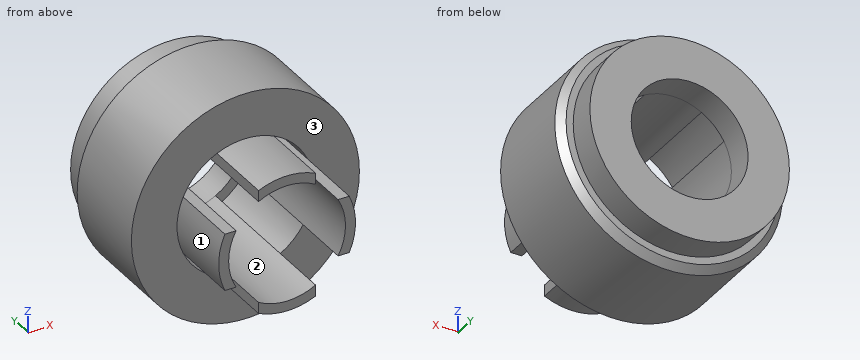
Autodesk Inventor part; units mm, degrees
ref_plane "YZ Plane" through (0, 0, 0) normal (1, 0, 0) x (0, 1, 0)
ref_plane "XZ Plane" through (0, 0, 0) normal (0, 1, 0) x (-1, 0, 0)
ref_plane "XY Plane" through (0, 0, 0) normal (0, 0, 1) x (1, 0, 0)
sketch "Sketch1" plane through (0, 0, 0) normal (0, 1, 0) x (-1, 0, 0)
  circle A0 centre (0, 0) radius 2.4
  circle A1 centre (0, 0) radius 4
  dimension "d0" = 8
  dimension "d1" = 4.8
extrude "Extrusion1" add sketch "Sketch1" along normal blind 3.5
chamfer "Chamfer1" distance 0.25 angle 45 1 edges at (4, 3.5, 0)
sketch "Sketch2" plane through (0, 3.5, 0) normal (0, 1, 0) x (1, 0, 0)
  circle A0 centre (0, 0) radius 2.05
  circle A1 centre (0, 0) radius 3.5
  dimension "d7" = 4.1
  dimension "d8" = 7
extrude "Extrusion2" add sketch "Sketch2" along normal blind 1
sketch "Sketch3" plane through (0, 3.5, 0) normal (0, -1, 0) x (1, 0, 0)
  arc A0 (-1.0733, -2.1466) -> (1, -2.1817) centre (0, 0) ccw
  arc A1 (-1, -1.7896) -> (1, -1.7896) centre (0, 0) ccw
  line L0 (-1, -1.7896) -> (-1, -2.1817)
  line L1 (1, -1.7896) -> (1, -2.1817)
  line L2 (0, 0) -> (0, -5.6159) construction
  dimension "d11" = 2.05
  dimension "d13" = 2.4
  dimension "d14" = 2
extrude "Extrusion3" add sketch "Sketch3" along normal blind 6
pattern_circular "Circular Pattern1" count 4 over 360 about axis through (0, -10, 0) along (0, 1, 0) of "Extrusion3"
properties part number "Collet" material "Acetal Resin, Black"
Part model, mm, in its own coordinate system. Face numbers are marked on the shaded views. A direction names the side the tool comes from. Coordinates: 2 decimals unless noted, no trailing zeros. Loops run counter-clockwise (first coordinate to the right, second up) from the corner with the lowest first, then second, coordinate; pieces in that order, holes last. Notation, with made-up numbers: M 45.5,81 L 70.5,81 A17 cw 70.5,87 Z; hole C 37,-19 d5. An arc over 180 degrees is marked long. Use a Markdown table: item, result. Add a question column.
Q1. Cut at A-A (y = -0.75). Write the cut outline in (x, z).
Q2. Pin check, flat tips, straight feed: P1, Ø1.5, axis at x = 3, y = 1, coming from the +Z side; P2, Ø2, axis at x = -1, y = 1, coming from the -Z side; P3, Ø0.9, axis at x = -1.5, z = 1.5, coming from the -Y side; P4, Ø1.5, axis at x = 0, y = -1.5, coming from the -Z side. Stop position of each tip, or through.
Q3. Cut at B-B (z = 0). Write the cut outline in (x, y), and give its area (3 significant figures).
Q4. Cut at C-C (x = 0). Write the cut outline in (y, z), and give its area (3 significant figures).
Q5. Probe L1, parallel to X at y = 4, z = 0; L2, parallel to X at y = -1.5, z = 0. List the from-to ranges inside material, lowest first.
Q6. Which spindle directions (+Z, -Z, +X, -X, +Y, -Y) get a long thin tool onto all of the face, cutting with end or side? Do the marked faces 1, 2 and 3. Say none if no direction does.
Q7. Cut at D-D (y = 1). Write the cut outline in (x, z), and give its area (3 significant figures).
Worked out:
| question | item | result |
|---|---|---|
| 1 | outline | M -2.18,-1 L -1.79,-1 A2.05 cw -1.79,1 L -2.18,1 A2.4 ccw Z; M -1,-2.18 A2.4 ccw 1,-2.18 L 1,-1.79 A2.05 cw -1,-1.79 Z; M -1,1.79 A2.05 cw 1,1.79 L 1,2.18 A2.4 ccw -1,2.18 Z; M 1.79,-1 L 2.18,-1 A2.4 ccw 2.18,1 L 1.79,1 A2.05 cw Z |
| 2 | P1 | stops at z = 3.31 |
| 2 | P2 | stops at z = -4 |
| 2 | P3 | stops at y = 0 |
| 2 | P4 | stops at z = -2.4 |
| 3 | outline | M -4,0 L -2.4,0 L -2.4,-2.5 L -2.05,-2.5 L -2.05,4.5 L -3.5,4.5 L -3.5,3.5 L -3.75,3.5 L -4,3.25 Z; M 2.05,-2.5 L 2.4,-2.5 L 2.4,0 L 4,0 L 4,3.25 L 3.75,3.5 L 3.5,3.5 L 3.5,4.5 L 2.05,4.5 Z |
| 3 | area | 18.2 mm2 |
| 4 | outline | M -2.5,-2.4 L 0,-2.4 L 0,-4 L 3.25,-4 L 3.5,-3.75 L 3.5,-3.5 L 4.5,-3.5 L 4.5,-2.05 L -2.5,-2.05 Z; M -2.5,2.05 L 4.5,2.05 L 4.5,3.5 L 3.5,3.5 L 3.5,3.75 L 3.25,4 L 0,4 L 0,2.4 L -2.5,2.4 Z |
| 4 | area | 18.2 mm2 |
| 5 | L1 | x = -3.5 to -2.05, 2.05 to 3.5 |
| 5 | L2 | x = -2.4 to -2.05, 2.05 to 2.4 |
| 6 | face 1 | -X, -Y |
| 6 | face 2 | +Y, -Y |
| 6 | face 3 | -Y |
| 7 | outline | C 0,0 d8; hole M -2.18,-1 A2.4 ccw -1,-2.18 L -1,-1.79 A2.05 ccw 1,-1.79 L 1,-2.18 A2.4 ccw 2.18,-1 L 1.79,-1 A2.05 ccw 1.79,1 L 2.18,1 A2.4 ccw 1,2.18 L 1,1.79 A2.05 ccw -1,1.79 L -1,2.18 A2.4 ccw -2.18,1 L -1.79,1 A2.05 ccw -1.79,-1 Z |
| 7 | area | 35.1 mm2 |
